Geometry check sheet. Reference: the model listing, model coordinates, mm. A direction names the side the tool comes from. Round coordinates to 2 decimals unless told otherwise and drop trailing zeros. Write each loop counter-clockwise with the first axis right and the second up, starting at its lowest first coordinate (ties: lowest second). Pieces come first, ordered by that corner, then holes. Notation, with made-up numbers: (48, 76) -> (105, 76) arc R7 cw to (105, 82) -> close; hole circle Ø3 at (80.5, 88.25). An arc over 180 degrees is marked (long way). Return JSON: item names as keys, results as strings. Group by question number.
from build123d import *

# Parameters (mm, degrees)
CUT_EXTRUDE3_DEPTH = 31.890937182
CIRPATTERN1_COUNT  = 4
CHAMFER1_SIZE      = 0.3


with BuildPart() as part:
    # Sketch1 → Revolve2 (revolve)
    with BuildSketch(Plane.XY, mode=Mode.PRIVATE) as revolve2_sk:
        with BuildLine():
            Line((17.605343981, 11), (17.605343981, 15))
            Line((17.605343981, 15), (6.305343981, 15))
            ThreePointArc((6.305343981, 15), (6.163922625, 15.058578644), (6.105343981, 15.2))
            Line((6.105343981, 15.2), (6.105343981, 18))
            Line((6.105343981, 18), (2.105343981, 18))
            Line((2.105343981, 18), (0.105343981, 16))
            Line((0.105343981, 16), (0.105343981, 11.1))
            ThreePointArc((0.105343981, 11.1), (0.3982372, 10.392893219), (1.105343981, 10.1))
            Line((1.105343981, 10.1), (4.605343981, 10.1))
            ThreePointArc((4.605343981, 10.1), (5.312450762, 9.807106781), (5.605343981, 9.1))
            Line((5.605343981, 9.1), (5.605343981, 4.6))
            Line((5.605343981, 4.6), (10.605343981, 4.6))
            Line((10.605343981, 4.6), (10.605343981, 11))
            Line((10.605343981, 11), (17.605343981, 11))
        make_face()
    revolve(revolve2_sk.sketch.rotate(Axis((0, 0, 0), (1, 0, 0)), 90), axis=Axis((0, 0, 0), (1, 0, 0)))

    # Sketch5 → Cut-Extrude3 (cut, through all)
    with BuildSketch(Plane.ZY.offset(-0.105343981)):
        with BuildLine():
            Line((0, 15), (0, 16))
            ThreePointArc((0, 16), (-1.253856039, 15.950794495), (-2.5, 15.803480629))
            Line((-2.5, 15.803480629), (-2.5, 15))
            Line((-2.5, 15), (0, 15))
        make_face()
        with BuildLine():
            ThreePointArc((2.5, 15.803480629), (1.253856039, 15.950794495), (0, 16))
            Line((0, 16), (0, 15))
            Line((0, 15), (2.5, 15))
            Line((2.5, 15), (2.5, 15.803480629))
        make_face()
        with BuildLine():
            Line((0, 18.508345056), (0, 18))
            Line((0, 18), (0, 16))
            ThreePointArc((0, 16), (1.253856039, 15.950794495), (2.5, 15.803480629))
            Line((2.5, 15.803480629), (2.5, 18.508345056))
            Line((2.5, 18.508345056), (0, 18.508345056))
        make_face()
        with BuildLine():
            Line((0, 16), (0, 18))
            Line((0, 18), (0, 18.508345056))
            Line((0, 18.508345056), (-2.5, 18.508345056))
            Line((-2.5, 18.508345056), (-2.5, 15.803480629))
            ThreePointArc((-2.5, 15.803480629), (-1.253856039, 15.950794495), (0, 16))
        make_face()
    cut_extrude3 = extrude(amount=-CUT_EXTRUDE3_DEPTH, mode=Mode.SUBTRACT)

    # CirPattern1: Cut-Extrude3 ×4 about axis
    cirpattern1_axis = Axis((0, 0, 0), (1, 0, 0))
    for i in range(1, CIRPATTERN1_COUNT):
        add(cut_extrude3.rotate(cirpattern1_axis, i * 360 / CIRPATTERN1_COUNT), mode=Mode.SUBTRACT)

    # Chamfer1
    chamfer1_edges = [part.edges().sort_by_distance(p)[0] for p in [
        (17.605343981, 0, -15),
    ]]
    chamfer(chamfer1_edges, length=CHAMFER1_SIZE)


solid = part.part
1) Sectioned sample at A-A on x = 8. Enter the section's corners in (y, z).
2) Tool access check on faces 1 (the face through (3, 0, 15)), 2 (the face through (3, -16, -2.5)), 3 (the face through (3, 16, 2.5)), 4 (the face through (3, 2.5, -16)). Record the directions out of +Z, -Z, +X, -X, +Y, -Y that give a thin tool (end or side, any length) a straight path to the whole face; none if there is none.
3) Mould release check, pull along Y, two halves, no side actions. Record for faces 5 (the face through (10.605, 5, 0)), 6 (the face through (3, -15, 0)), 7 (the face through (3, -16, 2.5)), 8 (the face through (14.15, 10.74, -2.38)): +Y half, -Y half, draft (parallel to the pull), parting line (faces both ways), or undercut.
4) Go/stop test with flat-tipped pins: P1, Ø1.5, axis at x = 3, z = 12.5, coming from the +Y side; P2, Ø1.5, axis at x = 4.5, z = 6.5, coming from the +Y side; P3, Ø3, axis at x = 5.5, z = -8.5, coming from the -Y side. Record where each tip stops, or that it passes through.
5) Material ranges on probe 1 along Y at (x, z) = (15.5, 0); probe 2 along Y at (x, z) = (8.15, 0); probe 3 along X at (y, z) = (4.5, 8), recorded low to high. Write a range as [from, to].
Evaluation:
{
 "1": {"outline": "circle Ø30 at (0, 0); hole circle Ø9.2 at (0, 0)"},
 "2": {"face 1": "+Z, +X, -X", "face 2": "+X, -X, -Y", "face 3": "+X, -X, +Y", "face 4": "-Z, +X, -X"},
 "3": {"face 5": "undercut", "face 6": "-Y half", "face 7": "draft", "face 8": "undercut"},
 "4": {"P1": "stops at y = 13.64", "P2": "stops at y = 17.06", "P3": "stops at y = -16.58"},
 "5": {"probe 1": "y = [-15, -11], [11, 15]", "probe 2": "y = [-15, -4.6], [4.6, 15]", "probe 3": "x = [5.6, 10.61]"}
}
